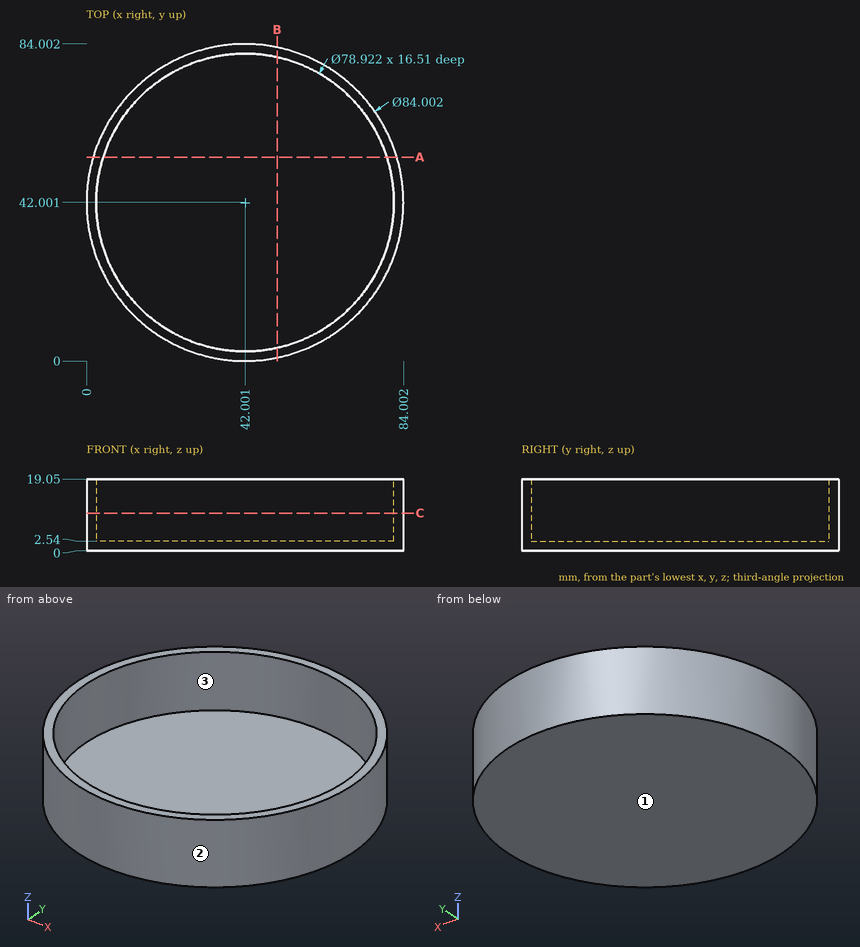
Design review of the part shown in the three views and the two pictorial views. Dimensions are in mm from the part's minimum x, y and z. Give positions to 0.01 mm unless a question says otherwise; leave off trailing zeros. Write each loop counter-clockwise with the first axis right and the second up, starting at its lowest first coordinate (ties: lowest second). Pieces come first, ordered by that corner, then holes. Notation, with made-up numbers: (-17, -38.5) -> (33, -38.5) arc R33 cw to (33, -3.5) -> close; hole circle Ø10 at (34.25, -12). An arc over 180 degrees is marked (long way). Answer in a Markdown table with one row per item.
1) For L1, parallel to Z at x = 46, y = 65.5; L2, parallel to Y at x = 56.5, z = 13; L3, parallel to Y at x = 17, z = 9.75, list the stretches that pass through material, from the lowest coordinate up. Write a range as [from, to].
Worked answers:
| item | result |
|---|---|
| L1 | [0, 2.54] |
| L2 | [2.58, 5.3], [78.7, 81.42] |
| L3 | [8.25, 11.47], [72.53, 75.75] |
2) Add section A-A on y = 54. State the section outline as (x, z) points.
Worked answers:
| item | result |
|---|---|
| outline | (1.75, 0) -> (82.25, 0) -> (82.25, 19.05) -> (79.59, 19.05) -> (79.59, 2.54) -> (4.41, 2.54) -> (4.41, 19.05) -> (1.75, 19.05) -> close |
3) Add section C-C on z = 10. State the section outline as (x, y) points, plus the area to 3 significant figures.
Worked answers:
| item | result |
|---|---|
| outline | circle Ø84 at (42, 42); hole circle Ø78.92 at (42, 42) |
| area | 650 mm² |
4) Clearance check with flat-ended pins moving along their axes: P1, Ø6, axis at x = 23.5, y = 43, coming from the +Z side; P2, Ø4, axis at x = 28.5, z = 7, coming from the +Y side; P3, Ø3, axis at x = 37, z = 8, coming from the +Y side. State where each tip first meets the part, or that it passes through.
Worked answers:
| item | result |
|---|---|
| P1 | z = 2.54 |
| P2 | y = 82.4 |
| P3 | y = 83.86 |
5) Mouldability with a two-part tool opening along X and no side actions: class the marked faces 1, 2 and 3 as +X half, -X half, draft (parallel to the pull), parting line (faces both ways), or undercut.
Worked answers:
| item | result |
|---|---|
| face 1 | draft |
| face 2 | parting line |
| face 3 | undercut |
6) Add section B-B on x = 50.5. State the section outline as (y, z) points.
Worked answers:
| item | result |
|---|---|
| outline | (0.87, 0) -> (83.13, 0) -> (83.13, 19.05) -> (80.54, 19.05) -> (80.54, 2.54) -> (3.47, 2.54) -> (3.47, 19.05) -> (0.87, 19.05) -> close |
